Read the model definition and answer for the solid it produces. Units are mm, in the model's axes. A direction names the side the tool comes from. Coordinates: 2 decimals unless noted, no trailing zeros. Loops run counter-clockwise (first coordinate to the right, second up) from the corner with the lowest first, then second, coordinate; pieces in that order, holes last. Notation, with made-up numbers: (48.25, 85.5) -> (72.25, 85.5) arc R23 ccw to (72.25, 93.5) -> close; hole circle Ø9 at (-22, 1.5). An arc over 180 degrees is marked (long way). Answer in a Markdown table with one row per item.
Autodesk Inventor part; units mm, degrees
ref_plane "YZ Plane" through (0, 0, 0) normal (1, 0, 0) x (0, 1, 0)
ref_plane "XZ Plane" through (0, 0, 0) normal (0, 1, 0) x (-1, 0, 0)
ref_plane "XY Plane" through (0, 0, 0) normal (0, 0, 1) x (1, 0, 0)
sketch "スケッチ1" plane through (0, 0, 0) normal (1, 0, 0) x (0, 1, 0)
  line L0 (0, -3.2) -> (0, 19.2) construction
  line L1 (-2.8, 0) -> (16.8, 0) construction
  line L2 (3, 16) -> (7.5, 16)
  line L3 (7.5, 16) -> (7.5, 4)
  line L4 (7.5, 4) -> (14, 4)
  line L5 (14, 4) -> (14, 0)
  line L6 (14, 0) -> (3, 0)
  line L7 (3, 0) -> (3, 16)
  point P0 (0, 0)
  dimension "d0" = 6
  dimension "d1" = 15
  dimension "d2" = 28
  dimension "d3" = 4
  dimension "d4" = 16
revolve "回転1" add sketch "スケッチ1" angle 360 about axis through (0, 0, -10) along (0, 0, 1)
sketch "スケッチ2" plane through (0, 0, 0) normal (1, 0, 0) x (0, 1, 0)
  line L0 (14, 0) -> (-14, 0) construction
  line L1 (0, -3.2) -> (0, 19.2) construction
  point P0 (0, 0)
  point P1 (0, 8)
  dimension "d8" = 8
hole "穴1" at (0, 0, 8) direction (1, 0, 0) diameter 3.242 end through all
sketch "スケッチ3" plane through (0, 0, 4) normal (0, 0, 1) x (1, 0, 0)
  circle A0 centre (-11.5, 0) radius 1.6
  line L0 (-19.6, 0) -> (19.6, 0) construction
  circle A1 centre (0, 0) radius 11.5 construction
  circle A2 centre (5.75, -9.9593) radius 1.6
  circle A3 centre (5.75, 9.9593) radius 1.6
  dimension "d16" = 23
  dimension "d17" = 3.2
  dimension "d20" = 360
extrude "押し出し1" cut sketch "スケッチ3" against normal through all
properties part number "mecanum_hub" material "アルミニウム 6061"
1. A cutting plane is placed at D-D on y = -9. Give the vertices of the cut face in (x, z).
A:
| item | result |
|---|---|
| outline | (-10.72, 0) -> (4.47, 0) -> (4.47, 4) -> (-10.72, 4) -> close; (7.03, 0) -> (10.72, 0) -> (10.72, 4) -> (7.03, 4) -> close |
2. Given pin 1 Ø4 at (x, y) = (-11.5, 0) entering from -Z; pin 2 Ø4 at (x, y) = (5.75, 9.96) entering from +Z; pin 3 Ø3 at (y, z) = (0, 8) entering from -X; pin 4 Ø4 at (x, z) = (3.5, 3.5) entering from +Y, each flat-ended and moving along its own axis, determine where each tip first touches the part or whether it passes through.
A:
| item | result |
|---|---|
| pin 1 | stops at z = 0 |
| pin 2 | stops at z = 4 |
| pin 3 | stops at x = -7.5 |
| pin 4 | stops at y = 13.92 |
3. A tool of negligible diameter and unlimited length cuts with its end or side. For faces 1 (the cylindrical face through (-5.362, 12.932, 1.972)), 2 (the flat face through (6, 6, 4)), from which of +Z, -Z, +X, -X, +Y, -Y can it reach the whole face along a straight path? Write none if from no direction.
A:
| item | result |
|---|---|
| face 1 | +Z, -Z |
| face 2 | +Z |
4. A cutting plane is placed at B-B on x = 0. Give the vertices of the cut face in (y, z), and give its area (3 significant figures).
A:
| item | result |
|---|---|
| outline | (-14, 0) -> (-3, 0) -> (-3, 16) -> (-7.5, 16) -> (-7.5, 4) -> (-14, 4) -> close; (3, 0) -> (14, 0) -> (14, 4) -> (7.5, 4) -> (7.5, 16) -> (3, 16) -> close |
| area | 196 mm2 |
5. A cutting plane is placed at C-C on y = 0. Give the vertices of the cut face in (x, z), and give its area (3 significant figures).
A:
| item | result |
|---|---|
| outline | (-14, 0) -> (-13.1, 0) -> (-13.1, 4) -> (-14, 4) -> close; (-9.9, 0) -> (-3, 0) -> (-3, 16) -> (-7.5, 16) -> (-7.5, 4) -> (-9.9, 4) -> close; (3, 0) -> (14, 0) -> (14, 4) -> (7.5, 4) -> (7.5, 6.38) -> (3, 6.38) -> close; (3, 9.62) -> (7.5, 9.62) -> (7.5, 16) -> (3, 16) -> close |
| area | 169 mm2 |
6. A cutting plane is placed at A-A on x = 5.75. Give the vertices of the cut face in (y, z).
A:
| item | result |
|---|---|
| outline | (-12.76, 0) -> (-11.56, 0) -> (-11.56, 4) -> (-12.76, 4) -> close; (-8.36, 0) -> (8.36, 0) -> (8.36, 4) -> (4.82, 4) -> (4.82, 16) -> (-4.82, 16) -> (-4.82, 4) -> (-8.36, 4) -> close; (11.56, 0) -> (12.76, 0) -> (12.76, 4) -> (11.56, 4) -> close; hole circle Ø3.24 at (0, 8) |
7. The mould has two halves that part along Y. Classify faces 3 (the flat face through (-3.3, -0.2, 0)), 4 (the cylindrical face through (5.542, -8.373, 2.028)), 5 (the cylindrical face through (5.05, -0.07, 6.38)), 6 (the cylindrical face through (-7.32, -1.63, 9.92)): pulls with the +Y half, pulls with the -Y half, needs draft (parallel to the pull), parting line crosses it, or undercut.
A:
| item | result |
|---|---|
| face 3 | needs draft |
| face 4 | undercut |
| face 5 | undercut |
| face 6 | parting line crosses it |
8. Find the intervals of material crossed by probe 1 along Y at (x, z) = (0, 3.25); probe 2 along Y at (x, z) = (7, 1.75); probe 3 along Y at (x, z) = (5.75, 2), in increasing order.
A:
| item | result |
|---|---|
| probe 1 | y = -14 to -3, 3 to 14 |
| probe 2 | y = -12.12 to -10.96, -8.96 to 8.96, 10.96 to 12.12 |
| probe 3 | y = -12.76 to -11.56, -8.36 to 8.36, 11.56 to 12.76 |
